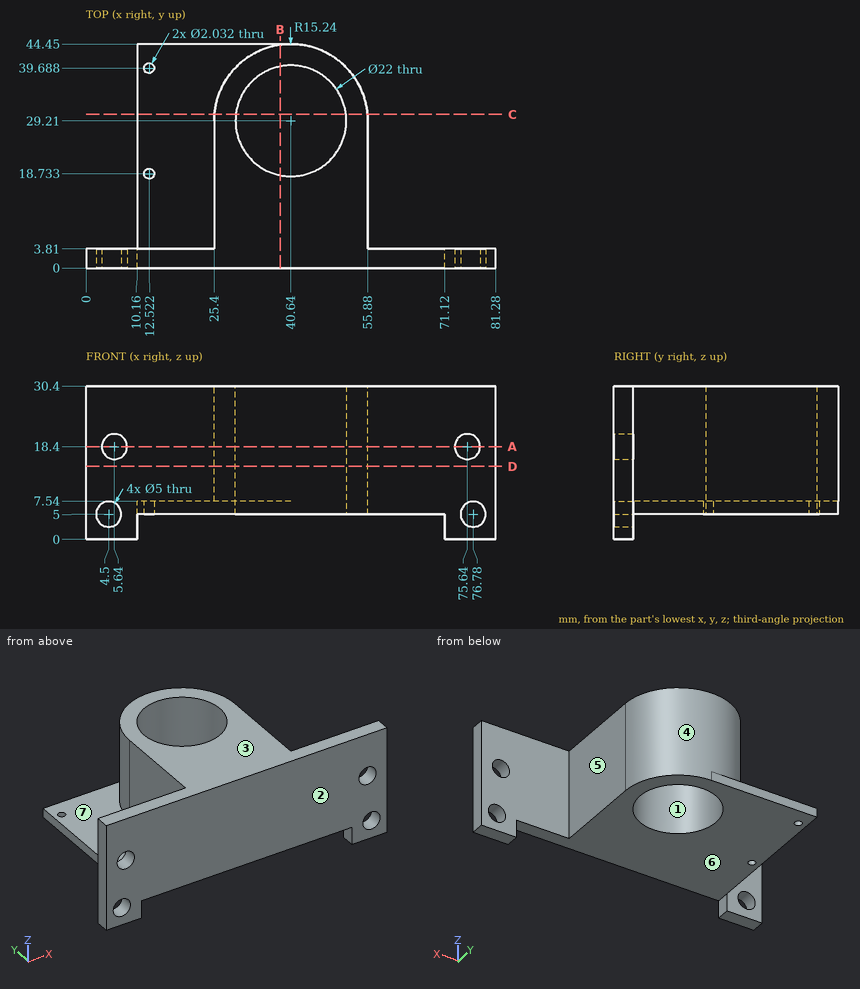
Geometry check sheet. Reference: drawing and pictorial views, mm from the part's lowest x, y, z. A direction names the side the tool comes from. Give positions to 0.01 mm unless a question says otherwise; leave off trailing zeros. Write each loop counter-clockwise with the first axis right and the second up, starting at its lowest first coordinate (ties: lowest second). Pieces come first, ordered by that corner, then holes. Notation, with made-up numbers: M 39.25,-4 L 63.25,-4 A16 ccw 63.25,23 Z; hole C -8,13 d2. An arc over 180 degrees is marked long. Put each result on its own line as item: value. Start each with the question number.
1. Go/stop test with flat-tipped pins: pin 1 Ø2 at (y, z) = (21, 22) entering from +X; pin 2 Ø6.5 at (x, z) = (4.5, 5) entering from +Y; pin 3 Ø12 at (x, z) = (18, 23) entering from -Y; pin 4 Ø2.5 at (x, y) = (12.52, 18.73) entering from -Z. Record where each tip stops, or that it passes through.
2. Scan lines: line 1 along X through (y, z) = (1.35, 18.4); line 2 along Z through (x, y) = (76, 2) (1 decimal); line 3 along X through (y, z) = (16.5, 24). Record each from-to range of solid material in increasing order. Write a range as [from, to].
3. Section check D-D (z = 14.5). Record the cut outline in (x, y).
4. Section check C-C (y = 30.5). Record the cut outline in (x, z) (1 decimal).
5. Section check A-A (z = 18.4). Record the cut outline in (x, y), and give its area (3 significant figures).
6. Draft check along Y on the marked faces 1, 2, 3 and 4. Enter one of: +Y half, -Y half, draft (parallel to the pull), parting line (faces both ways), or undercut.
7. Set-up check for the marked faces 5, 6 and 7: record each of +Z, -Z, +X, -X, +Y, -Y from which the full face is reachable in a straight line by a thin tool's end or side.
8. Section check B-B (x = 38.5). Record the cut outline in (y, z).
Answer list:
1. pin 1: x = 55.88
1. pin 2: y = 3.81
1. pin 3: y = 0
1. pin 4: z = 5
2. line 1: [0, 3.14], [8.14, 73.14], [78.14, 81.28]
2. line 2: [0, 2.6], [7.4, 15.9], [20.9, 30.4]
2. line 3: [25.4, 55.88]
3. outline: M 0,0 L 81.28,0 L 81.28,3.81 L 55.88,3.81 L 55.88,29.21 A15.24 ccw 25.4,29.21 L 25.4,3.81 L 0,3.81 Z; hole C 40.64,29.21 d22
4. outline: M 10.2,5 L 29.7,5 L 29.7,30.4 L 25.5,30.4 L 25.5,7.5 L 10.2,7.5 Z; M 51.6,5 L 55.8,5 L 55.8,30.4 L 51.6,30.4 Z
5. outline: M 0,0 L 3.14,0 L 3.14,3.81 L 0,3.81 Z; M 8.14,0 L 73.14,0 L 73.14,3.81 L 55.88,3.81 L 55.88,29.21 A15.24 ccw 25.4,29.21 L 25.4,3.81 L 8.14,3.81 Z; M 78.14,0 L 81.28,0 L 81.28,3.81 L 78.14,3.81 Z; hole C 40.64,29.21 d22
5. area: 1,030 mm2
6. face 1: undercut
6. face 2: -Y half
6. face 3: draft
6. face 4: +Y half
7. face 5: +Z, -Z, +X, +Y
7. face 6: -Z, +Y, -Y
7. face 7: +Z, -X, +Y
8. outline: M 0,5 L 18.42,5 L 18.42,30.4 L 0,30.4 Z; M 40,5 L 44.45,5 L 44.45,7.54 L 44.3,7.54 L 44.3,30.4 L 40,30.4 Z
